from build123d import *

# Parameters (mm, degrees)
F0_R     = 16
F0_R_2   = 2
F1_DEPTH = 1


with BuildPart() as f1:
    # F0 (on Front) → F1 (new body)
    with BuildSketch(Plane.XZ):
        with Locations((11.375166, 22.865392)):
            Circle(F0_R)
        with BuildLine():
            Line((4.209625, -1.647812), (4.209625, 1.420013))
            ThreePointArc((4.209625, 1.420013), (15.207091, 0.758549), (25.341338, 5.080448))
            Line((25.341338, 5.080448), (27.98607, 2.162959))
            ThreePointArc((27.98607, 2.162959), (33.227056, 2.037489), (33.08977, 7.27818))
            Line((33.08977, 7.27818), (30.211789, 9.875299))
            ThreePointArc((30.211789, 9.875299), (27.548758, 41.893357), (-4.572665, 42.57308))
            Line((-4.572665, 42.57308), (-8.227887, 46.289463))
            ThreePointArc((-8.227887, 46.289463), (-13.224062, 46.363974), (-13.364673, 41.369222))
            Line((-13.364673, 41.369222), (-11.350405, 39.209819))
            ThreePointArc((-11.350405, 39.209819), (-14.650167, 33.0315), (-15.790375, 26.12064))
            Line((-15.790375, 26.12064), (-15.790375, -1.647812))
            Line((-15.790375, -1.647812), (4.209625, -1.647812))
        make_face()
        with Locations((30.666229, 4.592549)):
            Circle(F0_R_2, mode=Mode.SUBTRACT)
        with Locations((11.375166, 22.865392)):
            Circle(F0_R, mode=Mode.SUBTRACT)
        with Locations((-10.763726, 43.795356)):
            Circle(F0_R_2, mode=Mode.SUBTRACT)
    extrude(amount=F1_DEPTH)


solid = f1.part
Work out the finished part from the listing and answer in its coordinate system (mm). A direction names the side the tool comes from. Coordinates: 2 decimals unless noted, no trailing zeros. Write each loop counter-clockwise with the first axis right and the second up, starting at its lowest first coordinate (ties: lowest second). Pieces come first, ordered by that corner, then holes. Notation, with made-up numbers: M 50.25,53 L 89.25,53 A25 cw 89.25,74 Z; hole C 81,34.25 d8. An arc over 180 degrees is marked long. Write item = value, one per line.
1. The part is cut by section C-C (y = -0.85). Determine the outline of the cut face in (x, z).
Solution:
outline = M -15.79,-1.65 L 4.21,-1.65 L 4.21,1.42 A24 ccw 25.34,5.08 L 27.99,2.16 A3.62 ccw long 33.09,7.28 L 30.21,9.88 A24 ccw -4.57,42.57 L -8.23,46.29 A3.56 ccw -13.36,41.37 L -11.35,39.21 A21.51 ccw -15.79,26.12 Z; hole C -10.76,43.8 d4; hole C 11.38,22.87 d32; hole C 30.67,4.59 d4
2. The part is cut by section A-A (z = 25). Determine the outline of the cut face in (x, y).
Solution:
outline = M -15.79,-1 L -4.48,-1 L -4.48,0 L -15.79,0 Z; M 27.23,-1 L 35.1,-1 L 35.1,0 L 27.23,0 Z
3. The part is cut by section D-D (z = 40). Determine the outline of the cut face in (x, y), then the cut area to 3 significant figures.
Solution:
outline = M -12.09,-1 L 29.35,-1 L 29.35,0 L -12.09,0 Z
area = 41.4 mm2
4. Determine the mould class of faces 4 (the face through (26.645, -0.493, 3.642)), 5 (the face through (-2, 0, 13)), 6 (the face through (-12.37, -0.49, 40.3)), 7 (the face through (-6.375, -0.493, 44.405)) for opening direction Z: released by +Z, released by -Z, zero draft, split by the parting line, or undercut.
Solution:
face_4 = released by -Z
face_5 = zero draft
face_6 = undercut
face_7 = released by +Z
5. Straight lines are drawn through the part: line 1 (X direction, y = -0.55, z = 43); line 2 (X direction, y = -0.75, z = 3); line 3 (X direction, y = -0.3, z = 42). For each, find the intervals that lie inside material, in ascending order. Write a range as from..to.
Solution:
line_1 = -14.23..-12.6, -8.93..-4.99, -4.06..26.29
line_2 = -15.79..21.96, 27.23..29.46, 31.88..33.91
line_3 = -13.83..-11.65, -9.88..27.43
6. A flat-ended cylindrical pin translates along its axis: pin 1 (4.5 mm diameter, centred on x = 30.67, z = 4.59, fed in from +Y). Find the tip coordinate at first contact, or state that the pin passes through.
Solution:
pin_1 = 0
7. For faces 1 (the face through (31.67, -0.49, 8.56)), 2 (the face through (29.079, -0.493, 3.376)), 3 (the face through (-14.62, -0.49, 33.12)), determine the directions among +Z, -Z, +X, -X, +Y, -Y from which every point of the face is accessible in a straight line to the end or side of a thin tool.
Solution:
face_1 = +X, +Y, -Y
face_2 = +Y, -Y
face_3 = -X, +Y, -Y
8. The part is cut by section B-B (x = -10). Determine the outline of the cut face in (y, z).
Solution:
outline = M -1,-1.65 L 0,-1.65 L 0,41.95 L -1,41.95 Z; M -1,45.64 L 0,45.64 L 0,47.27 L -1,47.27 Z
